```python
from build123d import *

# Parameters (mm, degrees)
SKETCH_1_W      = 20
SKETCH_1_H      = 20
EXTRUDE_1_DEPTH = 10
SKETCH_2_R      = 5
EXTRUDE_2_DEPTH = 10


with BuildPart() as part:
    # 草图1 → 凸台-拉伸1 (new body)
    with BuildSketch(Plane.XY):
        with Locations((10, -10)):
            Rectangle(SKETCH_1_W, SKETCH_1_H)
    extrude(amount=EXTRUDE_1_DEPTH)

    # 草图2 → 凸台-拉伸2 (add)
    with BuildSketch(Plane.ZY):
        with Locations((5, -5)):
            Circle(SKETCH_2_R)
    extrude(amount=EXTRUDE_2_DEPTH)


solid = part.part
```
Input: part model. Units: mm. Frame: model coordinates. A direction names the side the tool comes from. Coordinates: 2 decimals unless noted, no trailing zeros. Loops run counter-clockwise (first coordinate to the right, second up) from the corner with the lowest first, then second, coordinate; pieces in that order, holes last.
Q1. Line query: line 1 along X through (y, z) = (-15.5, 2.25); line 2 along Y through (x, z) = (-9, 5.25); line 3 along Y through (x, z) = (-2.5, 2.25). Output: solid intervals per line, ascending.
Results are:
line 1: x = 0 to 20
line 2: y = -9.99 to -0.01
line 3: y = -9.18 to -0.82
Q2. Set-up query: faces 1 (the flat face through (0, -1, 9)), 2 (the flat face through (10, -20, 5)), 3 (the flat face through (0, -1, 1)). Return all of +Z, -Z, +X, -X, +Y, -Y with unobstructed straight access to the full face (end or side cutting, diameter ignored); none if empty.
Results are:
face 1: +Z, -X, +Y
face 2: +Z, -Z, +X, -X, -Y
face 3: -Z, -X, +Y
Q3. Section B-B, the plane y = -14.5. Return the cut outline in (x, z), and give its area (3 significant figures).
Results are:
outline: (0, 0) - (20, 0) - (20, 10) - (0, 10) - close
area: 200 mm2
Q4. Section D-D, the plane z = 3. Return the cut outline in (x, y).
Results are:
outline: (-10, -9.58) - (0, -9.58) - (0, -20) - (20, -20) - (20, 0) - (0, 0) - (0, -0.42) - (-10, -0.42) - close
Q5. Section A-A, the plane z = 6.75. Return the cut outline in (x, y).
Results are:
outline: (-10, -9.68) - (0, -9.68) - (0, -20) - (20, -20) - (20, 0) - (0, 0) - (0, -0.32) - (-10, -0.32) - close
Q6. Mould query, pull axis X, two halves, no side actions, for faces 4 (the flat face through (20, -10, 5)), 5 (the cylindrical face through (-5, -8, 1)), 6 (the flat face through (-10, -5, 5)). Classes: +X half, -X half, draft (parallel to the pull), parting line (faces both ways), or undercut.
Results are:
face 4: +X half
face 5: draft
face 6: -X half
Q7. Section C-C, the plane x = -5.75. Return the cut outline in (y, z).
Results are:
outline: circle Ø10 at (-5, 5)
